```python
from build123d import *

# Parameters (mm, degrees)
SKETCH1_R           = 10
SKETCH1_R_2         = 3
SKETCH1_R_3         = 1.5
BOSS_EXTRUDE1_DEPTH = 5
SKETCH2_W           = 98.431457506
SKETCH2_H           = 81.46271096
SKETCH2_R           = 27.7
BOSS_EXTRUDE2_DEPTH = 13
SKETCH3_W           = 155
SKETCH3_H           = 81.46271096
SKETCH3_R           = 27.7
SKETCH3_R_2         = 1.2645
SKETCH3_R_3         = 4.5
BOSS_EXTRUDE3_DEPTH = 13
SKETCH4_R           = 18.5
SKETCH4_R_2         = 11
SKETCH4_R_3         = 1.2645
SKETCH4_R_4         = 4.5
CUT_EXTRUDE1_DEPTH  = 5
SKETCH4_3_R         = 11
SKETCH4_3_R_2       = 4.5
CUT_EXTRUDE2_DEPTH  = 8
LPATTERN1_COUNT     = 2
LPATTERN1_PITCH     = 104.6
CUT_EXTRUDE3_START  = -36
SKETCH5_W           = 23.598249953
SKETCH5_H           = 5
CUT_EXTRUDE3_DEPTH  = 23


with BuildPart() as part:
    # Sketch1 → Boss-Extrude1 (new body)
    with BuildSketch(Plane(origin=(0, 0, 0), x_dir=(1, 0, 0), z_dir=(0, 1, 0))):
        with BuildLine():
            Line((74.653701946, 78.479138322), (-74.346298054, 78.479138322))
            ThreePointArc((-74.346298054, 78.479138322), (-76.467618398, 77.600458666), (-77.346298054, 75.479138322))
            Line((-77.346298054, 75.479138322), (-77.346298054, -73.520861678))
            ThreePointArc((-77.346298054, -73.520861678), (-76.467618398, -75.642182022), (-74.346298054, -76.520861678))
            Line((-74.346298054, -76.520861678), (74.653701946, -76.520861678))
            ThreePointArc((74.653701946, -76.520861678), (76.775022289, -75.642182022), (77.653701946, -73.520861678))
            Line((77.653701946, -73.520861678), (77.653701946, 75.479138322))
            ThreePointArc((77.653701946, 75.479138322), (76.775022289, 77.600458666), (74.653701946, 78.479138322))
        make_face()
        with Locations((0.153701946, 34.979138322)):
            Circle(SKETCH1_R, mode=Mode.SUBTRACT)
        with Locations((68.153701946, -68.520861678)):
            Circle(SKETCH1_R_2, mode=Mode.SUBTRACT)
        with Locations((68.153701946, 70.479138322)):
            Circle(SKETCH1_R_2, mode=Mode.SUBTRACT)
        with Locations((-67.846298054, 70.479138322)):
            Circle(SKETCH1_R_2, mode=Mode.SUBTRACT)
        with Locations((-67.846298054, -68.520861678)):
            Circle(SKETCH1_R_2, mode=Mode.SUBTRACT)
        with Locations((-14.862359946, 14.189660085)):
            Circle(SKETCH1_R_3, mode=Mode.SUBTRACT)
        with Locations((-13.056819817, -14.03692357)):
            Circle(SKETCH1_R_3, mode=Mode.SUBTRACT)
        with Locations((15.169763838, -12.231383441)):
            Circle(SKETCH1_R_3, mode=Mode.SUBTRACT)
        with Locations((13.364223709, 15.995200214)):
            Circle(SKETCH1_R_3, mode=Mode.SUBTRACT)
    extrude(amount=-BOSS_EXTRUDE1_DEPTH)

    # Sketch2 → Boss-Extrude2 (add)
    with BuildSketch(Plane.XY.offset(66.520861678)):
        with Locations((0, -45.73135548)):
            Rectangle(SKETCH2_W, SKETCH2_H)
        with Locations((0, -47.5)):
            Circle(SKETCH2_R, mode=Mode.SUBTRACT)
    extrude(amount=-BOSS_EXTRUDE2_DEPTH)

    # Sketch3 → Boss-Extrude3 (add)
    with BuildSketch(Plane(origin=(0, 0, 3.020861678), x_dir=(-1, 0, 0), z_dir=(0, 0, -1))):
        with Locations((0, -45.73135548)):
            Rectangle(SKETCH3_W, SKETCH3_H)
        with Locations((0, -47.5)):
            Circle(SKETCH3_R, mode=Mode.SUBTRACT)
        with Locations((42.400505063, -57.399494937)):
            Circle(SKETCH3_R_2, mode=Mode.SUBTRACT)
        with Locations((42.400505063, -37.600505063)):
            Circle(SKETCH3_R_2, mode=Mode.SUBTRACT)
        with Locations((52.3, -47.5)):
            Circle(SKETCH3_R_3, mode=Mode.SUBTRACT)
        with Locations((62.199494937, -37.600505063)):
            Circle(SKETCH3_R_2, mode=Mode.SUBTRACT)
        with Locations((62.199494937, -57.399494937)):
            Circle(SKETCH3_R_2, mode=Mode.SUBTRACT)
        with Locations((-42.400505063, -57.390997892)):
            Circle(SKETCH3_R_2, mode=Mode.SUBTRACT)
        with Locations((-42.400505063, -37.592008019)):
            Circle(SKETCH3_R_2, mode=Mode.SUBTRACT)
        with Locations((-52.3, -47.5)):
            Circle(SKETCH3_R_3, mode=Mode.SUBTRACT)
        with Locations((-62.199494937, -57.390997892)):
            Circle(SKETCH3_R_2, mode=Mode.SUBTRACT)
        with Locations((-62.199494937, -37.592008019)):
            Circle(SKETCH3_R_2, mode=Mode.SUBTRACT)
    extrude(amount=BOSS_EXTRUDE3_DEPTH)

    # Sketch4 → Cut-Extrude1 (cut)
    with BuildSketch(Plane(origin=(0, 0, -9.979138322), x_dir=(-1, 0, 0), z_dir=(0, 0, -1))):
        with Locations((52.3, -47.5)):
            Circle(SKETCH4_R)
        with Locations((52.3, -47.5)):
            Circle(SKETCH4_R_2, mode=Mode.SUBTRACT)
        with Locations((62.199494937, -57.399494937)):
            Circle(SKETCH4_R_3, mode=Mode.SUBTRACT)
        with Locations((42.400505063, -57.399494937)):
            Circle(SKETCH4_R_3, mode=Mode.SUBTRACT)
        with Locations((62.199494937, -37.600505063)):
            Circle(SKETCH4_R_3, mode=Mode.SUBTRACT)
        with Locations((42.400505063, -37.600505063)):
            Circle(SKETCH4_R_3, mode=Mode.SUBTRACT)
        with Locations((52.3, -47.5)):
            Circle(SKETCH4_R_2)
        with Locations((52.3, -47.5)):
            Circle(SKETCH4_R_4, mode=Mode.SUBTRACT)
    cut_extrude1 = extrude(amount=-CUT_EXTRUDE1_DEPTH, mode=Mode.SUBTRACT)

    # Sketch4_3 → Cut-Extrude2 (cut)
    with BuildSketch(Plane(origin=(0, 0, -9.979138322), x_dir=(-1, 0, 0), z_dir=(0, 0, -1))):
        with Locations((52.3, -47.5)):
            Circle(SKETCH4_3_R)
        with Locations((52.3, -47.5)):
            Circle(SKETCH4_3_R_2, mode=Mode.SUBTRACT)
    cut_extrude2 = extrude(amount=-CUT_EXTRUDE2_DEPTH, mode=Mode.SUBTRACT)

    # LPattern1: Cut-Extrude1, Cut-Extrude2 ×2
    with Locations(*[(i * LPATTERN1_PITCH, 0, 0) for i in range(1, LPATTERN1_COUNT)]):
        add(cut_extrude1, mode=Mode.SUBTRACT)
        add(cut_extrude2, mode=Mode.SUBTRACT)

    # Sketch5 → Cut-Extrude3 (cut)
    with BuildSketch(Plane(origin=(0, 0, 0), x_dir=(1, 0, 0), z_dir=(0, 1, 0)).offset(CUT_EXTRUDE3_START)):
        with Locations((52.291592137, 7.479138322)):
            Rectangle(SKETCH5_W, SKETCH5_H)
    extrude(amount=-CUT_EXTRUDE3_DEPTH, mode=Mode.SUBTRACT)


solid = part.part
```
Geometry check sheet. Reference: the model listing, model coordinates, mm. A direction names the side the tool comes from. Round coordinates to 2 decimals unless told otherwise and drop trailing zeros. Loops run counter-clockwise (first coordinate to the right, second up) from the corner with the lowest first, then second, coordinate; pieces in that order, holes last. Notation, with made-up numbers: M -39.75,64.5 L 2.25,64.5 A13 cw 2.25,83.5 Z; hole C 62,14 d6. An arc over 180 degrees is marked long. Return JSON: item names as keys, results as strings. Group by question number.
(1) Section check A-A, the plane x = 52.3. Enter the section's corners in (y, z).
(2) Scan lines: line 1 along Z through (x, y) = (-36, -17); line 2 along Y through (x, z) = (52.5, -2.5); line 3 along Z through (x, y) = (44, -52.5). Record each from-to range of solid material in increasing order. Write a range as [from, to].
(3) Section check D-D, the plane x = 22. Enter the section's corners in (y, z).
(4) Section check C-C, the plane z = -42. Enter the section's corners in (x, y), and give its area (3 significant figures).
(5) Section check B-B, the plane y = -32.5. Enter the section's corners in (x, z).
(6) Mould release check, pull along Z, two halves, no side actions. Record for faces 4 (the face through (-1, -18, 53.521)), 5 (the face through (-1, -86.463, 60)), 6 (the face through (1, -2, -78.479)): pulls with the +Z half, pulls with the -Z half, needs draft (parallel to the pull), parting line crosses it, or undercut.
(7) Set-up check for faces 1 (the face through (-48.29, -65.56, -7.51)), 2 (the face through (1, -18, -9.979)), 3 (the face through (-1, -18, 66.521)): record each of +Z, -Z, +X, -X, +Y, -Y from which the full face is reachable in a straight line by a thin tool's end or side.
(8) Go/stop test with flat-tipped pins: pin 1 (3 mm diameter, centred on x = -62.2, y = -57.4, fed in from +Z); pin 2 (18.5 mm diameter, centred on x = 51, y = -53.5, fed in from -Z); pin 3 (3 mm diameter, centred on x = -27, z = 38, fed in from -Y); pin 4 (1.8 mm diameter, centred on x = -14.86, z = -14.19, fed in from +Y). Record where each tip stops, or that it passes through.
Data:
{
 "1": {"outline": "M -86.46,-9.98 L -66,-9.98 L -66,-4.98 L -58.5,-4.98 L -58.5,-1.98 L -52,-1.98 L -52,3.02 L -86.46,3.02 Z; M -43,-1.98 L -36.5,-1.98 L -36.5,-4.98 L -29,-4.98 L -29,-9.98 L -5,-9.98 L -5,-78.48 L 0,-78.48 L 0,76.52 L -5,76.52 L -5,3.02 L -43,3.02 Z"},
 "2": {"line 1": "[-9.98, 3.02], [53.52, 66.52]", "line 2": "[-86.46, -58.5], [-36.5, 0]", "line 3": "[-1.98, 3.02], [53.52, 66.52]"},
 "3": {"outline": "M -86.46,-9.98 L -64.33,-9.98 L -64.33,3.02 L -86.46,3.02 Z; M -86.46,53.52 L -64.33,53.52 L -64.33,66.52 L -86.46,66.52 Z; M -30.67,-9.98 L -5,-9.98 L -5,-78.48 L 0,-78.48 L 0,76.52 L -5,76.52 L -5,66.52 L -30.67,66.52 L -30.67,53.52 L -5,53.52 L -5,3.02 L -30.67,3.02 Z"},
 "4": {"outline": "M -77.35,-5 L -6.97,-5 L -6.97,0 L -77.35,0 Z; M 7.27,-5 L 77.65,-5 L 77.65,0 L 7.27,0 Z", "area": "704 mm²"},
 "5": {"outline": "M -77.5,-9.98 L -63.13,-9.98 L -63.13,-4.98 L -41.47,-4.98 L -41.47,-9.98 L -23.29,-9.98 L -23.29,3.02 L -77.5,3.02 Z; M -49.22,53.52 L -23.29,53.52 L -23.29,66.52 L -49.22,66.52 Z; M 23.29,-9.98 L 41.47,-9.98 L 41.47,-4.98 L 63.13,-4.98 L 63.13,-9.98 L 77.5,-9.98 L 77.5,3.02 L 23.29,3.02 Z; M 23.29,53.52 L 49.22,53.52 L 49.22,66.52 L 23.29,66.52 Z"},
 "6": {"face 4": "undercut", "face 5": "needs draft", "face 6": "pulls with the -Z half"},
 "7": {"face 1": "-Z", "face 2": "-Z, +X, -X, -Y", "face 3": "+Z, +X, -X, -Y"},
 "8": {"pin 1": "z = 3.02", "pin 2": "z = -4.98", "pin 3": "y = -5", "pin 4": "through"}
}
